from build123d import *
from build123d.topology import SkipClean

# Parameters (mm, degrees)
SKETCH3_R            = 4.15
BOSS_EXTRUDE2_DEPTH  = 10
FILLET1_R            = 4
BOSS_EXTRUDE3_START  = 42.5
BOSS_EXTRUDE3_DEPTH  = 42.5
FILLET1_OF_MIRROR1_R = 4
SKETCH5_W            = 20
SKETCH5_H            = 10
CUT_EXTRUDE1_DEPTH   = 10
SKETCH6_R            = 11
CUT_EXTRUDE2_DEPTH   = 10
SKETCH7_W            = 43
SKETCH7_H            = 43
CUT_EXTRUDE3_DEPTH   = 2
SKETCH8_R            = 1.55
CUT_EXTRUDE4_DEPTH   = 5
SKETCH9_W            = 10
SKETCH9_H            = 34.15
BOSS_EXTRUDE4_DEPTH  = 42.5
FILLET2_R            = 10
FILLET3_R            = 8
SKETCH10_R           = 4.15
BOSS_EXTRUDE5_DEPTH  = 10
SKETCH11_R           = 4.05
CUT_EXTRUDE5_DEPTH   = 77
FILLET4_R            = 25
FILLET5_R            = 4
FILLET6_R            = 4
SKETCH13_R           = 3.05
CUT_EXTRUDE6_DEPTH   = 12
SKETCH14_W           = 20
SKETCH14_H           = 4
BOSS_EXTRUDE6_DEPTH  = 42.5
FILLET7_R            = 2
SKETCH16_W           = 40
SKETCH16_H           = 40
CUT_EXTRUDE8_DEPTH   = 5
FILLET9_R            = 2
BOSS_EXTRUDE7_DEPTH  = 4
FILLET10_R           = 8
SKETCH18_R           = 2.55
CUT_EXTRUDE9_DEPTH   = 120.81756974
FILLET11_R           = 2


with BuildPart() as part:
    # Sketch3 → Boss-Extrude2 (new body)
    with BuildSketch(Plane(origin=(0, 0, 0), x_dir=(0, 0, -1), z_dir=(1, 0, 0))):
        Polygon((60, 0), (-100, 0), (-100, 20), (-50, 20), (-44.154765862, 44), (43.985309692, 44), align=None)
        with Locations((-30, 30)):
            Circle(SKETCH3_R, mode=Mode.SUBTRACT)
        with Locations(Location((30, 30, 0), (0, 0, 180))):
            Circle(SKETCH3_R, mode=Mode.SUBTRACT)
    boss_extrude2 = extrude(amount=BOSS_EXTRUDE2_DEPTH)

    # Fillet1
    fillet1_edges = [part.edges().sort_by_distance(p)[0] for p in [
        (5, 0, -60),
        (5, 0, 100),
        (5, 44, -43.985309692),
    ]]
    fillet(fillet1_edges, radius=FILLET1_R)

    # Sketch4 → Boss-Extrude3 (add)
    with BuildSketch(Plane.ZY.offset(BOSS_EXTRUDE3_START)):
        with BuildLine():
            Line((-34.995012035, 44), (-34.995012035, 34))
            Line((-34.995012035, 34), (-31.105667219, 34))
            ThreePointArc((-31.105667219, 34), (-30, 34.15), (-28.894332781, 34))
            Line((-28.894332781, 34), (28.894332781, 34))
            ThreePointArc((28.894332781, 34), (30, 34.15), (31.105667219, 34))
            Line((31.105667219, 34), (45.322569059, 34))
            Line((45.322569059, 34), (45.322569059, 39.205106235))
            Line((45.322569059, 39.205106235), (44.154765862, 44))
            Line((44.154765862, 44), (-34.995012035, 44))
        make_face()
    extrude(amount=-BOSS_EXTRUDE3_DEPTH)

    # Mirror1: Boss-Extrude2 across plane
    add(boss_extrude2.mirror(Plane.ZY.offset(21.25)))

    # Fillet1 of Mirror1
    fillet1_of_mirror1_edges = [part.edges().sort_by_distance(p)[0] for p in [
        (-47.5, 0, -60),
        (-47.5, 0, 100),
        (-47.5, 44, -43.985309692),
    ]]
    fillet(fillet1_of_mirror1_edges, radius=FILLET1_OF_MIRROR1_R)

    # Sketch5 → Cut-Extrude1 (cut)
    with SkipClean():  # the faces are left unmerged after this step: merging them gives an invalid solid
        with BuildSketch(Plane(origin=(10, 0, 0), x_dir=(0, 0, -1), z_dir=(1, 0, 0))):
            with Locations((0, 29)):
                Rectangle(SKETCH5_W, SKETCH5_H)
        extrude(amount=-CUT_EXTRUDE1_DEPTH, mode=Mode.SUBTRACT)

    # Sketch6 → Cut-Extrude2 (cut)
    with SkipClean():  # the faces are left unmerged after this step: merging them gives an invalid solid
        with BuildSketch(Plane.XZ.offset(-34)):
            with Locations(Location((-21.25, 0, 0), (0, 0, 270))):
                Circle(SKETCH6_R)
        extrude(amount=-CUT_EXTRUDE2_DEPTH, mode=Mode.SUBTRACT)

    # Sketch7 → Cut-Extrude3 (cut)
    with SkipClean():  # the faces are left unmerged after this step: merging them gives an invalid solid
        with BuildSketch(Plane(origin=(0, 44, 0), x_dir=(1, 0, 0), z_dir=(0, 1, 0))):
            with Locations((-21.25, 0)):
                Rectangle(SKETCH7_W, SKETCH7_H)
        extrude(amount=-CUT_EXTRUDE3_DEPTH, mode=Mode.SUBTRACT)

    # Sketch8 → Cut-Extrude4 (cut)
    with SkipClean():  # the faces are left unmerged after this step: merging them gives an invalid solid
        with BuildSketch(Plane(origin=(0, 42, 0), x_dir=(1, 0, 0), z_dir=(0, 1, 0))):
            with Locations(Location((-36.75, 15.5, 0), (0, 0, 270))):
                Circle(SKETCH8_R)
            with Locations(Location((-5.75, 15.5, 0), (0, 0, 90))):
                Circle(SKETCH8_R)
            with Locations(Location((-5.75, -15.5, 0), (0, 0, 270))):
                Circle(SKETCH8_R)
            with Locations(Location((-36.75, -15.5, 0), (0, 0, 90))):
                Circle(SKETCH8_R)
        extrude(amount=-CUT_EXTRUDE4_DEPTH, mode=Mode.SUBTRACT)

    # Sketch9 → Boss-Extrude4 (add)
    with SkipClean():  # the faces are left unmerged after this step: merging them gives an invalid solid
        with BuildSketch(Plane.ZY):
            with Locations((30, 17.075)):
                Rectangle(SKETCH9_W, SKETCH9_H)
        boss_extrude4 = extrude(amount=BOSS_EXTRUDE4_DEPTH)

    # Mirror2: Boss-Extrude4 across plane
    add(boss_extrude4.mirror(Plane(origin=(0, 0, 0), x_dir=(1, 0, 0), z_dir=(0, 0, -1))))

    # Fillet2
    fillet2_edges = [part.edges().sort_by_distance(p)[0] for p in [
        (0, 17, 35),
        (-42.5, 17, 35),
    ]]
    fillet(fillet2_edges, radius=FILLET2_R)

    # Fillet3
    fillet3_edges = [part.edges().sort_by_distance(p)[0] for p in [
        (0, 17.075, -35),
        (-42.5, 17.075, -35),
    ]]
    fillet(fillet3_edges, radius=FILLET3_R)

    # Sketch10 → Boss-Extrude5 (add)
    with BuildSketch(Plane.ZY.offset(52.5)):
        with Locations(Location((30, 30, 0), (0, 0, 180))):
            Circle(SKETCH10_R)
        with Locations((-30, 30)):
            Circle(SKETCH10_R)
    extrude(amount=-BOSS_EXTRUDE5_DEPTH)

    # Sketch11 → Cut-Extrude5 (cut)
    with BuildSketch(Plane(origin=(10, 0, 0), x_dir=(0, 0, -1), z_dir=(1, 0, 0))):
        with Locations((0, 10)):
            Circle(SKETCH11_R)
    extrude(amount=-CUT_EXTRUDE5_DEPTH, mode=Mode.SUBTRACT)

    # Fillet4
    fillet4_edges = [part.edges().sort_by_distance(p)[0] for p in [
        (5, 20, 50),
        (-47.5, 20, 50),
    ]]
    fillet(fillet4_edges, radius=FILLET4_R)

    # Fillet5
    fillet5_edges = [part.edges().sort_by_distance(p)[0] for p in [
        (5, 20, 100),
        (-47.5, 20, 100),
    ]]
    fillet(fillet5_edges, radius=FILLET5_R)

    # Fillet6
    fillet6_edges = [part.edges().sort_by_distance(p)[0] for p in [
        (-21.25, 44, 44.154765862),
    ]]
    fillet(fillet6_edges, radius=FILLET6_R)

    # Sketch13 → Cut-Extrude6 (cut)
    with BuildSketch(Plane(origin=(0, 44, 0), x_dir=(1, 0, 0), z_dir=(0, 1, 0))):
        with Locations(Location((5, -30, 0), (0, 0, 270))):
            Circle(SKETCH13_R)
        with Locations(Location((5, 30, 0), (0, 0, 270))):
            Circle(SKETCH13_R)
    extrude(amount=-CUT_EXTRUDE6_DEPTH, mode=Mode.SUBTRACT)

    # Sketch14 → Boss-Extrude6 (add)
    with BuildSketch(Plane(origin=(-42.5, 0, 0), x_dir=(0, 0, -1), z_dir=(1, 0, 0))):
        with Locations((-75, 2)):
            Rectangle(SKETCH14_W, SKETCH14_H)
    extrude(amount=BOSS_EXTRUDE6_DEPTH)

    # Fillet7
    fillet7_edges = [part.edges().sort_by_distance(p)[0] for p in [
        (0, 2, 65),
        (-42.5, 2, 65),
        (0, 2, 85),
        (-42.5, 2, 85),
    ]]
    fillet(fillet7_edges, radius=FILLET7_R)

    # Sketch16 → Cut-Extrude8 (cut)
    with BuildSketch(Plane(origin=(0, 34, 0), x_dir=(-1, 0, 0), z_dir=(0, -1, 0))):
        with Locations((21.25, 0)):
            Rectangle(SKETCH16_W, SKETCH16_H)
    extrude(amount=-CUT_EXTRUDE8_DEPTH, mode=Mode.SUBTRACT)

    # Fillet9
    fillet9_edges = [part.edges().sort_by_distance(p)[0] for p in [
        (0, 4, 75),
        (-42.5, 4, 75),
    ]]
    fillet(fillet9_edges, radius=FILLET9_R)

    # Sketch17 → Boss-Extrude7 (add)
    with BuildSketch(Plane(origin=(0, 0, 0), x_dir=(-1, 0, 0), z_dir=(0, -1, 0))):
        with BuildLine():
            Line((42.5, 48.643703987), (0, 48.643703987))
            Line((0, 48.643703987), (0, 43))
            ThreePointArc((0, 43), (2.343145751, 37.343145751), (8, 35))
            Line((8, 35), (34.5, 35))
            ThreePointArc((34.5, 35), (40.156854249, 37.343145751), (42.5, 43))
            Line((42.5, 43), (42.5, 48.643703987))
        make_face()
    extrude(amount=-BOSS_EXTRUDE7_DEPTH)

    # Fillet10
    fillet10_edges = [part.edges().sort_by_distance(p)[0] for p in [
        (0, 39.075, -34.995012035),
        (-42.5, 39.075, -34.995012035),
    ]]
    fillet(fillet10_edges, radius=FILLET10_R)

    # Sketch18 → Cut-Extrude9 (cut, through all)
    with BuildSketch(Plane(origin=(0, 4, 0), x_dir=(1, 0, 0), z_dir=(0, 1, 0))):
        with Locations(Location((-33.75, 42.143703987, 0), (0, 0, 270))):
            Circle(SKETCH18_R)
        with Locations(Location((-33.75, -75, 0), (0, 0, 270))):
            Circle(SKETCH18_R)
        with Locations(Location((-8.75, -75, 0), (0, 0, 90))):
            Circle(SKETCH18_R)
        with Locations(Location((-8.75, 42.143703987, 0), (0, 0, 90))):
            Circle(SKETCH18_R)
    extrude(amount=-CUT_EXTRUDE9_DEPTH, mode=Mode.SUBTRACT)

    # Fillet11
    fillet11_edges = [part.edges().sort_by_distance(p)[0] for p in [
        (-42.5, 4, -45.821851993),
        (-40.156854249, 4, -37.343145751),
        (-21.25, 4, -35),
        (-2.343145751, 4, -37.343145751),
        (0, 4, -45.821851993),
    ]]
    fillet(fillet11_edges, radius=FILLET11_R)


solid = part.part
Verification items for the finished model (mm, model axes). A direction names the side the tool comes from. Coordinates: 2 decimals unless noted, no trailing zeros. Order: outer loops, then holes, each group sorted by start corner. A loop starts at its lowest first (then second) coordinate and runs counter-clockwise, first axis right, second up.
1. Sectioned sample at B-B, the plane y = 10. Record the cut outline in (x, z).
Results found:
outline: (-52.5, -56.36) - (-42.5, -56.36) - (-42.5, -43) arc R8 cw to (-34.5, -35) - (-8, -35) arc R8 cw to (0, -43) - (0, -56.36) - (10, -56.36) - (10, -4.05) - (0, -4.05) - (0, -25) - (-42.5, -25) - (-42.5, -4.05) - (-52.5, -4.05) - close; (-52.5, 4.05) - (-42.5, 4.05) - (-42.5, 25) - (0, 25) - (0, 4.05) - (10, 4.05) - (10, 100) - (0, 100) - (0, 45) arc R10 cw to (-10, 35) - (-32.5, 35) arc R10 cw to (-42.5, 45) - (-42.5, 100) - (-52.5, 100) - close
2. Scan lines: line 1 (X direction, y = 10, z = 54); line 2 (Z direction, x = -33, y = 31); line 3 (Z direction, x = -33, y = 1). Record each from-to range of solid material in increasing order.
Results found:
line 1: x = -52.5 to -42.5, 0 to 10
line 2: z = -35 to -25, 25 to 35.01
line 3: z = -48.64 to -44.58, -39.71 to -25, 25 to 35.01, 65 to 72.56, 77.44 to 85
3. Set-up check for faces 1 (the face through (-2.281, 20.272, -37.406)), 2 (the face through (-21, 17, -25)), 3 (the face through (4.93, 25.95, 30.9)), 4 (the face through (-31, 42, -10)), 5 (the face through (5, 20, 83)): record each of +Z, -Z, +X, -X, +Y, -Y from which the full face is reachable in a straight line by a thin tool's end or side.
Results found:
face 1: -Z, +Y
face 2: -Y
face 3: +X
face 4: +Y
face 5: +Z, +X, -X, +Y
4. Sectioned sample at A-A, the plane z = 0. Give the number of separate pieces and of enclosed holes in the cut face, and give its area (3 significant figures).
Results found:
separate pieces: 5
enclosed holes: 0
area: 691 mm2
5. Go/stop test with flat-tipped pins: pin 1 Ø2.5 at (y, z) = (30.5, 30.5) entering from +X; pin 2 Ø12 at (x, z) = (-5.5, 26) entering from -Y; pin 3 Ø6 at (x, z) = (-25.5, 79.5) entering from +Y; pin 4 Ø4 at (x, z) = (-36.75, -15.5) entering from -Y. Record where each tip stops, or that it passes through.
Results found:
pin 1: stops at x = 0
pin 2: stops at y = 0
pin 3: stops at y = 4
pin 4: stops at y = 39
6. Release check for a two-part mould opening along Y. For faces 6 (the face through (-47.57, 1.141, 98.797)), 7 (the face through (0, 30, -30)), 8 (the face through (5.134, 38.485, 26.953)) record: +Y half, -Y half, draft (parallel to the pull), parting line (faces both ways), or undercut.
Results found:
face 6: -Y half
face 7: undercut
face 8: draft
